Verification items for the finished model (mm, model axes). A direction names the side the tool comes from. Coordinates: 2 decimals unless noted, no trailing zeros. Answer as a JSON object with one key per item and string values. Group by question number.
Q1. Release check for a two-part mould opening along Y. For faces 3 (the flat face through (-3.18, -26.35, 0.03)), 4 (the flat face through (-7, 1, 2.439)) record: released by +Y, released by -Y, zero draft, split by the parting line, or undercut.
Q2. Scan line: L1, parallel to X at y = 41.5, z = -0.7. Record every from-to range of solid material in increasing order.
Q3. Gauge pin test, flat ends, axial feed: pin 1 Ø0.5 at (y, z) = (-21.5, 0) entering from +X; pin 2 Ø1 at (x, z) = (-3.5, 0.5) entering from -Y. Record the tip position at first contact, or that the pin passes through.
Q4. Set-up check for faces 1 (the flat face through (-7, 1, -2.439)), 2 (the flat face through (-3.217, 10.728, 0.034)): record each of +Z, -Z, +X, -X, +Y, -Y from which the full face is reachable in a straight line by a thin tool's end or side.
```python
from build123d import *

# Parameters (mm, degrees)
RESSALTO_EXTRUS_O1_DEPTH = 5
SCALE2_SCALE             = 0.487804878


with BuildPart() as part:
    # Esboço1 → Ressalto-extrusão1 (new, symmetric)
    with BuildSketch(Plane.XY):
        Polygon((-2.596479089, -162.874745928), (2.546479089, -161.115750635), (2.546479089, -158.884249365), (-2.596479089, -157.125254072), (-2.596479089, -154.874745928), (2.546479089, -153.115750635), (2.546479089, -150.884249365), (-2.596479089, -149.125254072), (-2.596479089, -146.874745928), (2.546479089, -145.115750635), (2.546479089, -142.884249365), (-2.596479089, -141.125254072), (-2.596479089, -138.874745928), (2.546479089, -137.115750635), (2.546479089, -134.884249365), (-2.596479089, -133.125254072), (-2.596479089, -130.874745928), (2.546479089, -129.115750635), (2.546479089, -126.884249365), (-2.596479089, -125.125254072), (-2.596479089, -122.874745928), (2.546479089, -121.115750635), (2.546479089, -118.884249365), (-2.596479089, -117.125254072), (-2.596479089, -114.874745928), (2.546479089, -113.115750635), (2.546479089, -110.884249365), (-2.596479089, -109.125254072), (-2.596479089, -106.874745928), (2.546479089, -105.115750635), (2.546479089, -102.884249365), (-2.596479089, -101.125254072), (-2.596479089, -98.874745928), (2.546479089, -97.115750635), (2.546479089, -94.884249365), (-2.596479089, -93.125254072), (-2.596479089, -90.874745928), (2.546479089, -89.115750635), (2.546479089, -86.884249365), (-2.596479089, -85.125254072), (-2.596479089, -82.874745928), (2.546479089, -81.115750635), (2.546479089, -78.884249365), (-2.596479089, -77.125254072), (-2.596479089, -74.874745928), (2.546479089, -73.115750635), (2.546479089, -70.884249365), (-2.596479089, -69.125254072), (-2.596479089, -66.874745928), (2.546479089, -65.115750635), (2.546479089, -62.884249365), (-2.596479089, -61.125254072), (-2.596479089, -58.874745928), (2.546479089, -57.115750635), (2.546479089, -54.884249365), (-2.596479089, -53.125254072), (-2.596479089, -50.874745928), (2.546479089, -49.115750635), (2.546479089, -46.884249365), (-2.596479089, -45.125254072), (-2.596479089, -42.874745928), (2.546479089, -41.115750635), (2.546479089, -38.884249365), (-2.596479089, -37.125254072), (-2.596479089, -34.874745928), (2.546479089, -33.115750635), (2.546479089, -30.884249365), (-2.596479089, -29.125254072), (-2.596479089, -26.874745928), (2.546479089, -25.115750635), (2.546479089, -22.884249365), (-2.596479089, -21.125254072), (-2.596479089, -18.874745928), (2.546479089, -17.115750635), (2.546479089, -14.884249365), (-2.596479089, -13.125254072), (-2.596479089, -10.874745928), (2.546479089, -9.115750635), (2.546479089, -6.884249365), (-2.596479089, -5.125254072), (-2.596479089, -2.874745928), (2.546479089, -1.115750635), (2.546479089, 1.115750635), (-2.596479089, 2.874745928), (-2.596479089, 5.125254072), (2.546479089, 6.884249365), (2.546479089, 9.115750635), (-2.596479089, 10.874745928), (-2.596479089, 13.125254072), (2.546479089, 14.884249365), (2.546479089, 17.115750635), (-2.596479089, 18.874745928), (-2.596479089, 21.125254072), (2.546479089, 22.884249365), (2.546479089, 25.115750635), (-2.596479089, 26.874745928), (-2.596479089, 29.125254072), (2.546479089, 30.884249365), (2.546479089, 33.115750635), (-2.596479089, 34.874745928), (-2.596479089, 37.125254072), (2.546479089, 38.884249365), (2.546479089, 41.115750635), (-2.596479089, 42.874745928), (-2.596479089, 45.125254072), (2.546479089, 46.884249365), (2.546479089, 49.115750635), (-2.596479089, 50.874745928), (-2.596479089, 53.125254072), (2.546479089, 54.884249365), (2.546479089, 57.115750635), (-2.596479089, 58.874745928), (-2.596479089, 61.125254072), (2.546479089, 62.884249365), (2.546479089, 65.115750635), (-2.596479089, 66.874745928), (-2.596479089, 69.125254072), (2.546479089, 70.884249365), (2.546479089, 73.115750635), (-2.596479089, 74.874745928), (-2.596479089, 77.125254072), (2.546479089, 78.884249365), (2.546479089, 81.115750635), (-2.596479089, 82.874745928), (-2.596479089, 85.125254072), (2.546479089, 86.884249365), (2.546479089, 89.115750635), (-2.596479089, 90.874745928), (-2.596479089, 93.125254072), (2.546479089, 94.884249365), (2.546479089, 97.115750635), (-2.596479089, 98.874745928), (-2.596479089, 101.125254072), (2.546479089, 102.884249365), (2.546479089, 105.115750635), (-2.596479089, 106.874745928), (-2.596479089, 109.125254072), (2.546479089, 110.884249365), (2.546479089, 113.115750635), (-2.596479089, 114.874745928), (-2.596479089, 117.125254072), (2.546479089, 118.884249365), (2.546479089, 121.115750635), (-2.596479089, 122.874745928), (-2.596479089, 125.125254072), (2.546479089, 126.884249365), (2.546479089, 129.115750635), (-2.596479089, 130.874745928), (-2.596479089, 133.125254072), (2.546479089, 134.884249365), (2.546479089, 137.115750635), (-2.596479089, 138.874745928), (-2.596479089, 141.125254072), (2.546479089, 142.884249365), (2.546479089, 145.115750635), (-2.596479089, 146.874745928), (-2.596479089, 149.125254072), (2.546479089, 150.884249365), (2.546479089, 153.115750635), (-2.596479089, 154.874745928), (-2.596479089, 157.125254072), (2.546479089, 158.884249365), (2.546479089, 161.115750635), (-2.596479089, 162.874745928), (-2.596479089, 164), (-12.782395447, 164), (-12.782395447, -164), (-2.596479089, -164), align=None)
    extrude(amount=RESSALTO_EXTRUS_O1_DEPTH, both=True)


with BuildPart() as part_1:
    # Scale2: scaled about (-6.22348049, 0, 0)
    add(part.part.scale(SCALE2_SCALE).moved(Location((-3.187636349, 0, 0))))


solid = part_1.part
```
Computed values:
{
 "1": {"face 3": "undercut", "face 4": "zero draft"},
 "2": {"L1": "x = -9.42 to -4.45"},
 "3": {"pin 1": "stops at x = -4.45", "pin 2": "stops at y = -79.3"},
 "4": {"face 1": "-Z, +X, -X, +Y, -Y", "face 2": "+Z, -Z, +X"}
}
